Geometry check sheet. Reference: the model listing, model coordinates, mm. A direction names the side the tool comes from. Round coordinates to 2 decimals unless told otherwise and drop trailing zeros. Order: outer loops, then holes, each group sorted by start corner. A loop starts at its lowest first (then second) coordinate and runs counter-clockwise, first axis right, second up. Notation, with made-up numbers: (16.25, -3.75) -> (36.25, -3.75) arc R20 ccw to (36.25, 35.25) -> close; hole circle Ø2 at (13, 84). An arc over 180 degrees is marked (long way). Use a Markdown table: item, result. Add a question column.
Item 1: Sectioned sample at D-D, the plane z = 15. Record the cut outline in (x, y).
Item 2: Set-up check for faces 1 (the flat face through (-120, -34, 1)), 2 (the flat face through (45, -54, 1)): record each of +Z, -Z, +X, -X, +Y, -Y from which the full face is reachable in a straight line by a thin tool's end or side.
Item 3: Sectioned sample at A-A, the plane z = 40. Record the cut outline in (x, y), and give its area (3 significant figures).
Item 4: Sectioned sample at B-B, the plane y = -81. Record the cut outline in (x, z).
Item 5: Material ranges on probe 1 along X at (y, z) = (-23, 0); probe 2 along X at (y, z) = (-63.5, 0); probe 3 along Z at (x, y) = (-58, -44.5), recorded low to high. Write a range as [from, to].
Item 6: Gauge pin test, flat ends, axial feed: pin 1 Ø4 at (x, z) = (10.5, -67.5) entering from +Y; pin 2 Ø10 at (x, y) = (-44, -36) entering from -Z; pin 3 Ø6 at (x, y) = (56, -39.5) entering from -Z; pin 4 Ø4 at (x, z) = (60.5, 45) entering from -Y. Record the tip position at first contact, or that the pin passes through.
Item 7: Mould release check, pull along X, two halves, no side actions. Record for faces 3 (the cylindrical face through (81.975, -50.988, -1.121)), 4 (the cylindrical face through (-21.48, -43.88, 42.92)), 5 (the flat face through (120, -19, -1)): pulls with the +X half, pulls with the -X half, needs draft (parallel to the pull), parting line crosses it, or undercut.
Item 8: Sectioned sample at C-C, the plane x = -35. Record the cut outline in (y, z).
from build123d import *

# Parameters (mm, degrees)
SCHIZZO1_W                   = 165
SCHIZZO1_H                   = 178
ESTRUSIONE_ESTRUSIONE3_DEPTH = 89
TAGLIO_ESTRUSIONE1_DEPTH     = 208.525901998
ESTRUSIONE_ESTRUSIONE5_DEPTH = 75
SCHIZZO6_R                   = 45
TAGLIO_ESTRUSIONE2_DEPTH     = 174.902271406


with BuildPart() as part:
    # Schizzo1 → Estrusione-Estrusione3 (new body)
    with BuildSketch(Plane(origin=(0, 0, 0), x_dir=(1, 0, 0), z_dir=(0, 1, 0))):
        with Locations((-37.5, 0)):
            Rectangle(SCHIZZO1_W, SCHIZZO1_H)
    extrude(amount=-ESTRUSIONE_ESTRUSIONE3_DEPTH)

    # Schizzo3 → Taglio-Estrusione1 (cut, through all)
    with BuildSketch(Plane(origin=(45, 0, 0), x_dir=(0, 0, -1), z_dir=(1, 0, 0))):
        with BuildLine():
            Line((89, -89), (89, 0))
            ThreePointArc((89, 0), (62.932503523, -62.932503528), (-7e-09, -89))
            Line((-7e-09, -89), (89, -89))
        make_face()
        with BuildLine():
            ThreePointArc((-7e-09, -89), (-62.932503528, -62.932503523), (-89, 0))
            Line((-89, 0), (-89, -89))
            Line((-89, -89), (-7e-09, -89))
        make_face()
    extrude(amount=-TAGLIO_ESTRUSIONE1_DEPTH, mode=Mode.SUBTRACT)

    # Schizzo4 → Estrusione-Estrusione5 (add)
    with BuildSketch(Plane(origin=(45, 0, 0), x_dir=(0, 0, -1), z_dir=(1, 0, 0))):
        with BuildLine():
            Line((-51, 0), (51, 0))
            ThreePointArc((51, 0), (0, -51), (-51, 0))
        make_face()
    extrude(amount=ESTRUSIONE_ESTRUSIONE5_DEPTH)

    # Schizzo6 → Taglio-Estrusione2 (cut, through all)
    with BuildSketch(Plane(origin=(0, 0, 0), x_dir=(1, 0, 0), z_dir=(0, 1, 0))):
        with Locations(Location((-35, 0, 0), (0, 0, 270))):
            Circle(SCHIZZO6_R)
    extrude(amount=-TAGLIO_ESTRUSIONE2_DEPTH, mode=Mode.SUBTRACT)


solid = part.part
Found:
| question | item | result |
|---|---|---|
| 1 | outline | (-120, -87.73) -> (-77.43, -87.73) -> (-77.43, 0) -> (-120, 0) -> close; (7.43, -87.73) -> (45, -87.73) -> (45, -48.74) -> (120, -48.74) -> (120, 0) -> (7.43, 0) -> close |
| 2 | face 1 | +Z, -Z, -X, +Y, -Y |
| 2 | face 2 | +X, -Y |
| 3 | outline | (-120, -79.5) -> (-55.62, -79.5) -> (-55.62, 0) -> (-120, 0) -> close; (-14.38, -79.5) -> (45, -79.5) -> (45, -31.64) -> (120, -31.64) -> (120, 0) -> (-14.38, 0) -> close |
| 3 | area | 12,200 mm2 |
| 4 | outline | (-120, -36.88) -> (-60.79, -36.88) arc R45 cw to (-60.79, 36.88) -> (-120, 36.88) -> close; (-9.21, -36.88) -> (45, -36.88) -> (45, 36.88) -> (-9.21, 36.88) arc R45 cw to start |
| 5 | probe 1 | x = [-120, -80], [10, 120] |
| 5 | probe 2 | x = [-120, -80], [10, 45] |
| 5 | probe 3 | z = [-77.08, -38.68], [38.68, 77.08] |
| 6 | pin 1 | stops at y = 0 |
| 6 | pin 2 | stops at z = -83.43 |
| 6 | pin 3 | stops at z = -35.62 |
| 6 | pin 4 | stops at y = -27.42 |
| 7 | face 3 | needs draft |
| 7 | face 4 | undercut |
| 7 | face 5 | pulls with the +X half |
| 8 | outline | (-76.79, -45) arc R89 ccw to (0, -89) -> (0, -45) -> close; (-76.79, 45) -> (0, 45) -> (0, 89) arc R89 ccw to start |
